Study the drawing (mm; zero at the part's minimum x, y, z) and answer. A direction names the side the tool comes from. Round coordinates to 2 decimals unless told otherwise and drop trailing zeros. Write each loop counter-clockwise with the first axis right and the second up, starting at its lowest first coordinate (ties: lowest second). Pieces come first, ordered by that corner, then holes.
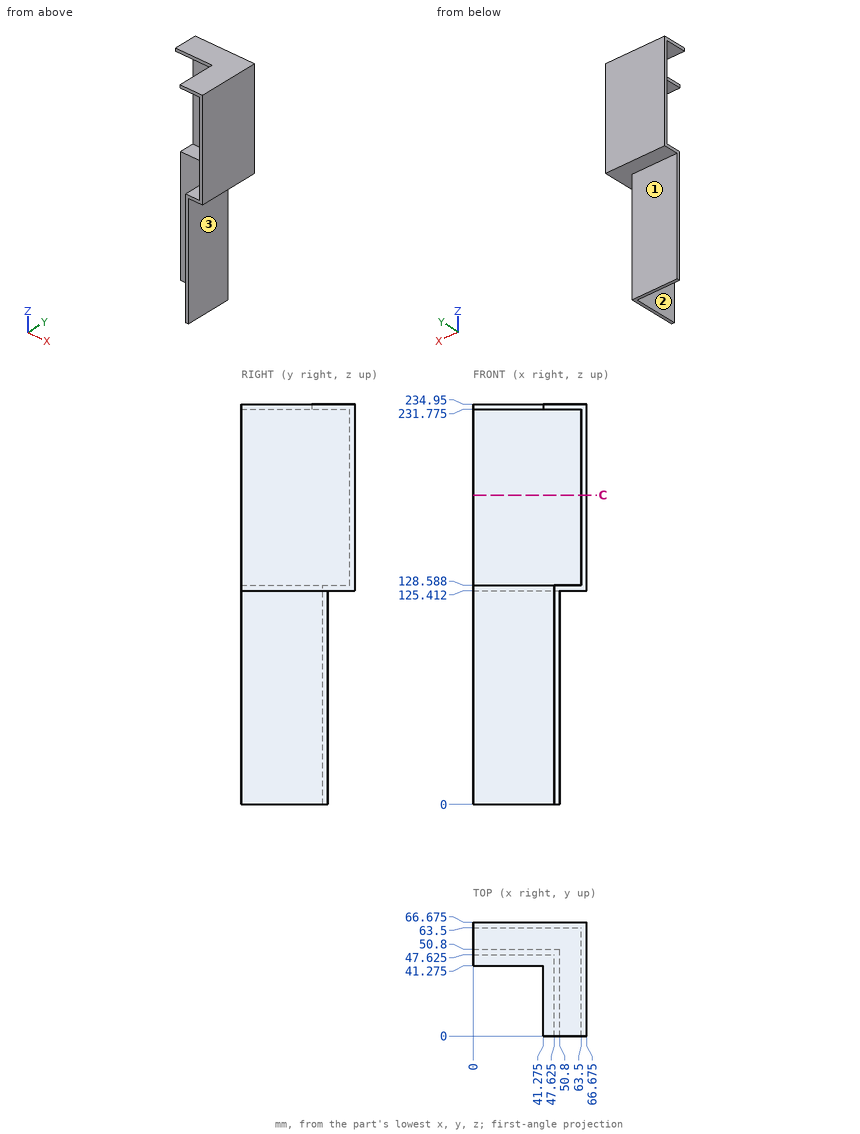
Q1. Find section C-C (z = 181.5). Determine the outline of the cut face in (x, y) (1 decimal).
Q2. Find the intervals of material crossed by L1, parallel to X at y = 42, z = 46 (1 decimal); L2, parallel to Y at x = 51, z = 174.5 (1 decimal), in increasing order.
Q3. A tool of negligible diameter and unlimited length cuts with its end or side. For the marked faces 1, 2 and 3, from which of +Z, -Z, +X, -X, +Y, -Y can it reach the whole face along a straight path? Write none if from no direction.
Q4. Given pin 1 (1 mm diameter, centred on y = 8, z = 176.5, fed in from -X); pin 2 (1.6 mm diameter, centred on y = 23, z = 234, fed in from -X) (1 decimal); pin 3 (10 mm diameter, centred on x = 58, z = 68, fed in from +Y); pin 4 (2.5 mm diameter, centred on x = 30, z = 234, fed in from -Y) (1 decimal), each flat-ended and moving along its own axis, determine where each tip first touches the part or whether it passes through.
Report:
1. outline: (0, 63.5) - (63.5, 63.5) - (63.5, 0) - (66.7, 0) - (66.7, 66.7) - (0, 66.7) - close
2. L1: x = 47.6 to 50.8
2. L2: y = 63.5 to 66.7
3. face 1: -Z, +X, -X, +Y
3. face 2: -Z, -X, -Y
3. face 3: -Z, +X, +Y, -Y
4. pin 1: stops at x = 63.5
4. pin 2: stops at x = 41.3
4. pin 3: passes through
4. pin 4: stops at y = 41.3
